Could you check a few things on this model? Use its own coordinates, in mm. A direction names the side the tool comes from. Round coordinates to 2 decimals unless told otherwise and drop trailing zeros. Write each loop counter-clockwise with the first axis right and the second up, starting at its lowest first coordinate (ties: lowest second). Pieces come first, ordered by that corner, then holes. Notation, with made-up numbers: (62, -29.5) -> (86, -29.5) arc R35 cw to (86, 3.5) -> close; hole circle Ø2 at (-19, -25.75). An arc over 180 degrees is marked (long way). Answer as CSV lines item,"result". Start each with the question number.
Q1. If we mould it in two halves opening along X, with no side actions, what happens to faces 3 (the flat face through (-7, 11, 1)), 4 (the cylindrical face through (-33.592, 12.601, -1.028)), 5 (the flat face through (30.5, 0, -1))? For each: pulls with the +X half, pulls with the -X half, needs draft (parallel to the pull), parting line crosses it, or undercut.
Q2. For faces 1 (the cylindrical face through (29.9, 15.43, -0.97)), 2 (the flat face through (-34, 1, -1)), which set-ups out of +Z, -Z, +X, -X, +Y, -Y let a thin tool reach every point of the face, with its end or its side?
Q3. Imagine slicing it at A-A on x = -35.5. Please give me the cut outline in (y, z), and give its area (3 significant figures).
Q4. Imagine slicing it at C-C on x = 20.5. Please give me the cut outline in (y, z).
Q5. Imagine slicing it at D-D on x = -15.5. Please give me the cut outline in (y, z), and give its area (3 significant figures).
Q6. Imagine slicing it at B-B on y = 5. Please give me the cut outline in (x, z).
Q7. If I drill on line 1 (Y direction, x = -35.5, z = -0.95); line 2 (Y direction, x = 20.5, z = -1.7); line 3 (Y direction, x = -13.5, z = -0.2), over which ranges is the centre line in solid material (lowest first)? Write a range as [from, to].
from build123d import *

# Parameters (mm, degrees)
SKETCH007_W = 73
SKETCH007_H = 32
SKETCH007_R = 2
PAD_DEPTH   = 4
FILLET_R    = 0.6
FILLET001_R = 1
FILLET002_R = 0.6
FILLET003_R = 2


with BuildPart() as part:
    # Sketch007 → Pad (new body)
    with BuildSketch(Plane.XY.offset(-3)):
        with Locations((-6, 0)):
            Rectangle(SKETCH007_W, SKETCH007_H)
        with Locations((-35.5, 5)):
            Circle(SKETCH007_R, mode=Mode.SUBTRACT)
        with Locations((-35.5, -5)):
            Circle(SKETCH007_R, mode=Mode.SUBTRACT)
        with Locations((13.5, 5)):
            Circle(SKETCH007_R, mode=Mode.SUBTRACT)
        with Locations((13.5, -5)):
            Circle(SKETCH007_R, mode=Mode.SUBTRACT)
        with Locations((-35.5, 12)):
            Circle(SKETCH007_R, mode=Mode.SUBTRACT)
        with Locations((-35.5, -12)):
            Circle(SKETCH007_R, mode=Mode.SUBTRACT)
        with Locations((20.5, 12)):
            Circle(SKETCH007_R, mode=Mode.SUBTRACT)
        with Locations((20.5, -12)):
            Circle(SKETCH007_R, mode=Mode.SUBTRACT)
        with Locations((26.5, -12)):
            Circle(SKETCH007_R, mode=Mode.SUBTRACT)
        with Locations((26.5, 12)):
            Circle(SKETCH007_R, mode=Mode.SUBTRACT)
        Polygon((-31, 10.5), (9, 10.5), (9, 1), (15, 1), (15, -1), (9, -1), (9, -10.5), (-31, -10.5), (-31, -1), (-37, -1), (-37, 1), (-31, 1), align=None, mode=Mode.SUBTRACT)
    extrude(amount=PAD_DEPTH)

    # Fillet
    fillet_edges = [part.edges().sort_by_distance(p)[0] for p in [
        (9, -10.5, -1),
        (9, 10.5, -1),
        (-31, 10.5, -1),
        (-31, -10.5, -1),
    ]]
    fillet(fillet_edges, radius=FILLET_R)

    # Fillet001
    fillet001_edges = [part.edges().sort_by_distance(p)[0] for p in [
        (-31, -1, -1),
        (-31, 1, -1),
        (9, -1, -1),
        (9, 1, -1),
    ]]
    fillet(fillet001_edges, radius=FILLET001_R)

    # Fillet002
    fillet002_edges = [part.edges().sort_by_distance(p)[0] for p in [
        (-37, -1, -1),
        (-37, 1, -1),
        (15, -1, -1),
        (15, 1, -1),
    ]]
    fillet(fillet002_edges, radius=FILLET002_R)

    # Fillet003
    fillet003_edges = [part.edges().sort_by_distance(p)[0] for p in [
        (30.5, 16, -1),
        (30.5, -16, -1),
        (-42.5, 16, -1),
        (-42.5, -16, -1),
    ]]
    fillet(fillet003_edges, radius=FILLET003_R)


solid = part.part
Checks:
1,face 3,"needs draft"
1,face 4,"undercut"
1,face 5,"pulls with the +X half"
2,face 1,"+Z, -Z, +X, +Y"
2,face 2,"+Z, -Z"
3,outline,"(-16, -3) -> (-14, -3) -> (-14, 1) -> (-16, 1) -> close; (-10, -3) -> (-7, -3) -> (-7, 1) -> (-10, 1) -> close; (-3, -3) -> (-1, -3) -> (-1, 1) -> (-3, 1) -> close; (1, -3) -> (3, -3) -> (3, 1) -> (1, 1) -> close; (7, -3) -> (10, -3) -> (10, 1) -> (7, 1) -> close; (14, -3) -> (16, -3) -> (16, 1) -> (14, 1) -> close"
3,area,"56.0 mm^2"
4,outline,"(-16, -3) -> (-14, -3) -> (-14, 1) -> (-16, 1) -> close; (-10, -3) -> (10, -3) -> (10, 1) -> (-10, 1) -> close; (14, -3) -> (16, -3) -> (16, 1) -> (14, 1) -> close"
5,outline,"(-16, -3) -> (-10.5, -3) -> (-10.5, 1) -> (-16, 1) -> close; (10.5, -3) -> (16, -3) -> (16, 1) -> (10.5, 1) -> close"
5,area,"44.0 mm^2"
6,outline,"(-42.5, -3) -> (-37.5, -3) -> (-37.5, 1) -> (-42.5, 1) -> close; (-33.5, -3) -> (-31, -3) -> (-31, 1) -> (-33.5, 1) -> close; (9, -3) -> (11.5, -3) -> (11.5, 1) -> (9, 1) -> close; (15.5, -3) -> (30.5, -3) -> (30.5, 1) -> (15.5, 1) -> close"
7,line 1,"[-16, -14], [-10, -7], [-3, -1], [1, 3], [7, 10], [14, 16]"
7,line 2,"[-16, -14], [-10, 10], [14, 16]"
7,line 3,"[-16, -10.5], [10.5, 16]"
